```python
from build123d import *

# Parameters (mm, degrees)
BOSS_EXTRUDE1_DEPTH             = 10
CUT_EXTRUDE1_START              = -6
CUT_EXTRUDE1_DEPTH              = 4
CBORE_FOR_M6_SHCS1_D            = 6.6
CBORE_FOR_M6_SHCS1_CBORE_D      = 11
CBORE_FOR_M6_SHCS1_CBORE_DEPTH  = 6
F_4_0MM_CLEARANCE_DOWEL_HOLE1_D = 4


with BuildPart() as part:
    # Sketch2 → Boss-Extrude1 (new body)
    with BuildSketch(Plane.XY):
        with BuildLine():
            Line((-23, 47), (14, 47))
            ThreePointArc((14, 47), (15.414213562, 46.414213562), (16, 45))
            Line((16, 45), (16, -18))
            ThreePointArc((16, -18), (15.414213562, -19.414213562), (14, -20))
            Line((14, -20), (-23, -20))
            ThreePointArc((-23, -20), (-24.414213562, -19.414213562), (-25, -18))
            Line((-25, -18), (-25, 45))
            ThreePointArc((-25, 45), (-24.414213562, 46.414213562), (-23, 47))
        make_face()
        with BuildLine():
            Line((-4.06, 22), (-4.06, 5))
            ThreePointArc((-4.06, 5), (0, 0.94), (4.06, 5))
            Line((4.06, 5), (4.06, 22))
            ThreePointArc((4.06, 22), (0, 26.06), (-4.06, 22))
        make_face(mode=Mode.SUBTRACT)
    extrude(amount=-BOSS_EXTRUDE1_DEPTH)

    # Sketch3 → Cut-Extrude1 (cut)
    with BuildSketch(Plane.XY.offset(CUT_EXTRUDE1_START)):
        with BuildLine():
            Line((-5.06, 22), (-5.06, 5))
            ThreePointArc((-5.06, 5), (0, -0.06), (5.06, 5))
            Line((5.06, 5), (5.06, 22))
            ThreePointArc((5.06, 22), (0, 27.06), (-5.06, 22))
        make_face()
    extrude(amount=-CUT_EXTRUDE1_DEPTH, mode=Mode.SUBTRACT)

    # CBORE for M6 SHCS1 (through all)
    with Locations(Plane(origin=(0, 0, 0), x_dir=(0.9063077870366375, -0.4226182617407263, 0), z_dir=(0, 0, 1))):
        with Locations((-30.560418539, 27.67780372), (10.992955388, -7.011057825), (-9.852123713, -16.731277845), (-9.715339437, 37.39802374)):
            CounterBoreHole(CBORE_FOR_M6_SHCS1_D / 2, CBORE_FOR_M6_SHCS1_CBORE_D / 2, CBORE_FOR_M6_SHCS1_CBORE_DEPTH)

    # Ø4.0mm Clearance Dowel Hole1 (through all)
    with Locations(Plane(origin=(0, 0, 0), x_dir=(0.9063077870366375, -0.4226182617407263, 0), z_dir=(0, 0, 1))):
        with Locations((-18.294727782, 34.500767171), (-1.272735368, -13.834021277)):
            Hole(F_4_0MM_CLEARANCE_DOWEL_HOLE1_D / 2)


solid = part.part
```
Source: CAD feature listing. Evaluate the final solid. Frame: model axes, mm. A direction names the side the tool comes from. Give positions to 0.01 mm unless a question says otherwise; leave off trailing zeros. Loops run counter-clockwise (first coordinate to the right, second up) from the corner with the lowest first, then second, coordinate; pieces in that order, holes last. Notation, with made-up numbers: M 36.25,52 L 68.25,52 A20 ccw 68.25,85 Z; hole C -35,69.5 d9. An arc over 180 degrees is marked long. Put each result on its own line as item: value.
Q1. Section A-A (x = -16). Return the cut outline in (y, z), and give its area (3 significant figures).
Response values:
outline: M -20,-10 L -14.3,-10 L -14.3,-6 L -16.5,-6 L -16.5,0 L -20,0 Z; M -7.7,-10 L 34.7,-10 L 34.7,-6 L 32.5,-6 L 32.5,0 L -5.5,0 L -5.5,-6 L -7.7,-6 Z; M 41.3,-10 L 47,-10 L 47,0 L 43.5,0 L 43.5,-6 L 41.3,-6 Z
area: 485 mm²
Q2. Section D-D (y = -12). Return the cut outline in (x, z).
Response values:
outline: M -25,-10 L -19.14,-10 L -19.14,-6 L -21.41,-6 L -21.41,0 L -25,0 Z; M -12.86,-10 L -9,-10 L -9,0 L -10.59,0 L -10.59,-6 L -12.86,-6 Z; M -5,-10 L 3.86,-10 L 3.86,-6 L 1.59,-6 L 1.59,0 L -5,0 Z; M 10.14,-10 L 16,-10 L 16,0 L 12.41,0 L 12.41,-6 L 10.14,-6 Z
Q3. Mould query, pull axis X, two halves, no side actions, for faces 1 (the cylindrical face through (15.4, 46.43, -4.93)), 2 (the cylindrical face through (-18.103, 43.082, -2.958)), 3 (the flat face through (-25, 13, -5)), 4 (the flat face through (-9, 14, -10)). Classes: released by +X, released by -X, zero draft, split by the parting line, or undercut.
Response values:
face 1: released by +X
face 2: undercut
face 3: released by -X
face 4: zero draft
Q4. Section C-C (z = -8). Return the cut outline in (x, y).
Response values:
outline: M -25,-18 A2 ccw -23,-20 L 14,-20 A2 ccw 16,-18 L 16,45 A2 ccw 14,47 L -23,47 A2 ccw -25,45 Z; hole C -16,-11 d6.6; hole C -16,38 d6.6; hole C -7,-12 d4; hole M -5.06,5 A5.06 ccw 5.06,5 L 5.06,22 A5.06 ccw -5.06,22 Z; hole C -2,39 d4; hole C 7,-11 d6.6; hole C 7,38 d6.6
Q5. Section B-B (x = -7). Return the cut outline in (y, z).
Response values:
outline: M -20,-10 L -14,-10 L -14,0 L -20,0 Z; M -10,-10 L 47,-10 L 47,0 L -10,0 Z
Q6. Pin query (flat end, axial travel): P1, Ø10, axis at x = 7, y = 38, coming from the +Z side; P2, Ø6, axis at x = 7, y = 38, coming from the -Z side. Return the tip coordinate at first contact, or that it passes through.
Response values:
P1: stops at z = -6
P2: passes through
Q7. Reachability of faces 5 (the flat face through (-12.7, -12.4, -6)), 6 (the cylindrical face through (0.09, 26.06, -2.96)), 7 (the flat face through (5.06, 13, -8)) from +Z, -Z, +X, -X, +Y, -Y: full face, straight path, thin tool, end or side. Return the list, or none.
Response values:
face 5: +Z
face 6: +Z, -Z
face 7: -Z
Q8. Line query: probe 1 along X at (y, z) = (-11, -7.7); probe 2 along Y at (x, z) = (10, -4); probe 3 along Y at (x, z) = (-16, -2.2). Output: solid intervals per line, ascending. Write a range as [from, to].
Response values:
probe 1: x = [-25, -19.3], [-12.7, -8.73], [-5.27, 3.7], [10.3, 16]
probe 2: y = [-20, -15.61], [-6.39, 33.39], [42.61, 47]
probe 3: y = [-20, -16.5], [-5.5, 32.5], [43.5, 47]
